```python
from build123d import *

# Parameters (mm, degrees)
SKETCH_1_W          = 20
SKETCH_1_H          = 13
SKETCH_1_R          = 0.8
EXTRUDE_1_DEPTH     = 2
SKETCH_2_W          = 20
SKETCH_2_H          = 44
EXTRUDE_2_DEPTH     = 2
SKETCH_3_R          = 8
SKETCH_3_R_2        = 4.5
EXTRUDE_3_DEPTH     = 10
SKETCH_4_R          = 20
EXTRUDE_4_DEPTH     = 2
SKETCH_6_W          = 20.177677641
SKETCH_6_H          = 1.475
CUT_EXTRUDE_1_DEPTH = 4
FILLET_1_R          = 3


with BuildPart() as part:
    # 草图1 → 凸台-拉伸1 (new body)
    with BuildSketch(Plane.XY):
        with Locations((10, -6.5)):
            Rectangle(SKETCH_1_W, SKETCH_1_H)
        with Locations((10, -2.8)):
            Circle(SKETCH_1_R, mode=Mode.SUBTRACT)
        with Locations((17, -9.8)):
            Circle(SKETCH_1_R, mode=Mode.SUBTRACT)
        with Locations((3, -9.8)):
            Circle(SKETCH_1_R, mode=Mode.SUBTRACT)
    extrude_1 = extrude(amount=EXTRUDE_1_DEPTH)

    # 草图2 → 凸台-拉伸2 (add)
    with BuildSketch(Plane(origin=(0, 0, 0), x_dir=(1, 0, 0), z_dir=(0, 1, 0))):
        with Locations((10, -22)):
            Rectangle(SKETCH_2_W, SKETCH_2_H)
    extrude(amount=EXTRUDE_2_DEPTH)

    # 镜向1: 凸台-拉伸1 across plane
    add(extrude_1.mirror(Plane.XY.offset(22)))

    # 草图3 → 凸台-拉伸3 (add)
    with BuildSketch(Plane(origin=(0, 2, 0), x_dir=(1, 0, 0), z_dir=(0, 1, 0))):
        with Locations((10, -22)):
            Circle(SKETCH_3_R)
        with Locations((10, -22)):
            Circle(SKETCH_3_R_2, mode=Mode.SUBTRACT)
    extrude(amount=EXTRUDE_3_DEPTH)

    # 草图4 → 凸台-拉伸4 (add)
    with BuildSketch(Plane(origin=(0, 2, 0), x_dir=(1, 0, 0), z_dir=(0, 1, 0))):
        with Locations((10, -22)):
            Circle(SKETCH_4_R)
    extrude(amount=-EXTRUDE_4_DEPTH)

    # 草图6 → 切除-旋转1 (revolve, cut)
    with BuildSketch(Plane(origin=(0, 5.5, 0), x_dir=(1, 0, 0), z_dir=(0, 1, 0))):
        with Locations((10.210002175, -21.25904805)):
            Rectangle(SKETCH_6_W, SKETCH_6_H)
    revolve(axis=Axis((22.976612399, 5.5, 21.99654805), (-1, 0, 0)), mode=Mode.SUBTRACT)

    # 草图7 → 切除-拉伸1 (cut)
    with BuildSketch(Plane.XY.offset(34)):
        Polygon((9.704672539, 4.57882911), (9.704672539, 2), (9.704672539, 1.881120606), (9.704672539, -0.127173503), (10.704672539, -0.127173503), (10.704672539, 4.57882911), align=None)
    extrude(amount=-CUT_EXTRUDE_1_DEPTH, mode=Mode.SUBTRACT)

    # 圆角1
    fillet_1_edges = [part.edges().sort_by_distance(p)[0] for p in [
        (0, -13, 43),
        (20, -13, 43),
        (20, -13, 1),
        (0, -13, 1),
    ]]
    fillet(fillet_1_edges, radius=FILLET_1_R)


solid = part.part
```
The model under review builds one solid part; all positions refer to its coordinate system, in mm. A direction names the side the tool comes from. Round coordinates to 2 decimals unless told otherwise and drop trailing zeros. Loops run counter-clockwise (first coordinate to the right, second up) from the corner with the lowest first, then second, coordinate; pieces in that order, holes last. Notation, with made-up numbers: (5, 18) - (23, 18) arc R20 cw to (23, 41) - close; hole circle Ø3 at (70, -23.5). An arc over 180 degrees is marked (long way). Use a Markdown table: item, result. Add a question column.
Q1. Add section A-A (y = -2.8). State the section outline as (x, z) points.
Q2. Add section D-D (z = 20). State the section outline as (x, y) points.
Q3. Machinability: for faces 1 (the face through (10, -5, 44)), 2 (the face through (10, 1, 34)), 3 (the face through (17.39, 6.93, 25.06)), 4 (the face through (10, -6, 42)), which of the approach directions +Z, -Z, +X, -X, +Y, -Y give a long, thin tool a straight path to every point of the face, cutting with its end or side? Answer none if there is none.
Q4. Insertion check: pin 1 Ø1 at (x, z) = (21, 29) entering from -Y; pin 2 Ø12 at (x, z) = (22.5, 6) entering from +Y; pin 3 Ø2.5 at (y, z) = (-2.5, 3) entering from +X. Each pin has a flat end and moves straight along its axis. Give the tip position at first contact, or say it passes through.
Q5. Add section B-B (y = -6.75). State the section outline as (x, z) points.
Q6. The part is to be moulded in two halves that separate along X. For faces 5 (the face through (10, -13, 43)), 6 (the face through (14.16, 6.93, 23.72)), 7 (the face through (0.86, -12.1, 1.01)), say which applies: pulls with the +X half, pulls with the -X half, needs draft (parallel to the pull), parting line crosses it, or undercut.
Q7. For probe 1 along Z at (x, y) = (14, -9); probe 2 along Y at (x, z) = (22, 36); probe 3 along Z at (x, y) = (3.9, 5.5), list the stretches that pass through material, from the lowest coordinate up.
Q8. Add section C-C (y = 8). State the section outline as (x, z) points, plus the area to 3 significant figures.
Worked answers:
| question | item | result |
|---|---|---|
| 1 | outline | (0, 0) - (9.2, 0) - (9.2, 2) - (0, 2) - close; (0, 42) - (9.2, 42) - (9.2, 44) - (0, 44) - close; (10.8, 0) - (20, 0) - (20, 2) - (10.8, 2) - close; (10.8, 42) - (20, 42) - (20, 44) - (10.8, 44) - close |
| 2 | outline | (-9.9, 0) - (29.9, 0) - (29.9, 2) - (17.75, 2) - (17.75, 12) - (14.03, 12) - (14.03, 2) - (5.97, 2) - (5.97, 12) - (2.25, 12) - (2.25, 2) - (-9.9, 2) - close |
| 3 | face 1 | +Z, +X, -X, +Y, -Y |
| 3 | face 2 | +Y, -Y |
| 3 | face 3 | +Y |
| 3 | face 4 | +X, -X, -Y |
| 4 | pin 1 | y = 0 |
| 4 | pin 2 | y = 2 |
| 4 | pin 3 | x = 20 |
| 5 | outline | (0, 0) - (20, 0) - (20, 2) - (0, 2) - close; (0, 42) - (20, 42) - (20, 44) - (0, 44) - close |
| 6 | face 5 | needs draft |
| 6 | face 6 | undercut |
| 6 | face 7 | pulls with the -X half |
| 7 | probe 1 | 0 to 2, 42 to 44 |
| 7 | probe 2 | 0 to 2 |
| 7 | probe 3 | 16.82 to 20.52, 23.47 to 27.18 |
| 8 | outline | circle Ø16 at (10, 22); hole circle Ø9 at (10, 22) |
| 8 | area | 137 mm² |
